from build123d import *

# Parameters (mm, degrees)
SKETCH1_R           = 37.5
BOSS_EXTRUDE1_DEPTH = 55
SKETCH2_R           = 16
CUT_EXTRUDE1_DEPTH  = 16
SKETCH3_R           = 16
CUT_EXTRUDE2_DEPTH  = 2.5
SKETCH6_R           = 8.9296875
CUT_EXTRUDE3_DEPTH  = 12.7
CUT_EXTRUDE4_START  = -15.35
SKETCH7_R           = 37.5
CUT_EXTRUDE4_DEPTH  = 15.35
SKETCH9_R           = 3.302
CUT_EXTRUDE6_DEPTH  = 67.216482087
BOSS_EXTRUDE2_START = 10
SKETCH10_R          = 37.5
SKETCH10_R_2        = 8.9296875
SKETCH10_R_3        = 3.302
BOSS_EXTRUDE2_DEPTH = 10


with BuildPart() as part:
    # Sketch1 → Boss-Extrude1 (new body)
    with BuildSketch(Plane.XY):
        Circle(SKETCH1_R)
    extrude(amount=BOSS_EXTRUDE1_DEPTH)

    # Sketch2 → Cut-Extrude1 (cut)
    with BuildSketch(Plane.XY.offset(55)):
        Circle(SKETCH2_R)
    extrude(amount=-CUT_EXTRUDE1_DEPTH, mode=Mode.SUBTRACT)

    # Sketch3 → Cut-Extrude2 (cut)
    with BuildSketch(Plane.XY.offset(39)):
        Circle(SKETCH3_R)
    extrude(amount=-CUT_EXTRUDE2_DEPTH, mode=Mode.SUBTRACT)

    # Sketch4 → Cut-Revolve1 (revolve, cut)
    with BuildSketch(Plane(origin=(0, 0, 0), x_dir=(0, 0, -1), z_dir=(1, 0, 0))):
        with BuildLine():
            Line((-12.7, 8.9281), (-12.7, 0))
            Line((-12.7, 0), (-36.5, 0))
            Line((-36.5, 0), (-36.5, 12))
            add(Edge.make_bspline(
                [(-36.5, 12), (-28.343745376, 16.523417527), (-19.165864626, 14.261468976), (-12.7, 8.9281)],
                knots=[0, 0, 0, 0, 1, 1, 1, 1], degree=3))
        make_face()
    revolve(axis=Axis((0, 0, 12.7), (0, 0, 1)), mode=Mode.SUBTRACT)

    # Sketch6 → Cut-Extrude3 (cut)
    with BuildSketch(Plane(origin=(0, 0, 0), x_dir=(-1, 0, 0), z_dir=(0, 0, -1))):
        Circle(SKETCH6_R)
    extrude(amount=-CUT_EXTRUDE3_DEPTH, mode=Mode.SUBTRACT)

    # Sketch7 → Cut-Extrude4 (cut)
    with BuildSketch(Plane.XY.offset(55).offset(CUT_EXTRUDE4_START)):
        Circle(SKETCH7_R)
    extrude(amount=CUT_EXTRUDE4_DEPTH, mode=Mode.SUBTRACT)

    # Sketch9 → Cut-Extrude6 (cut, through all)
    with BuildSketch(Plane(origin=(0, 0, 0), x_dir=(-1, 0, 0), z_dir=(0, 0, -1))):
        with Locations((0, -27.5)):
            Circle(SKETCH9_R)
        with Locations((-19.445436483, -19.445436483)):
            Circle(SKETCH9_R)
        with Locations((-27.5, 0)):
            Circle(SKETCH9_R)
        with Locations((-19.445436483, 19.445436483)):
            Circle(SKETCH9_R)
        with Locations((0, 27.5)):
            Circle(SKETCH9_R)
        with Locations((19.445436483, 19.445436483)):
            Circle(SKETCH9_R)
        with Locations((27.5, 0)):
            Circle(SKETCH9_R)
        with Locations((19.445436483, -19.445436483)):
            Circle(SKETCH9_R)
    extrude(amount=-CUT_EXTRUDE6_DEPTH, mode=Mode.SUBTRACT)

    # Sketch10 → Boss-Extrude2 (add)
    with BuildSketch(Plane(origin=(0, 0, 0), x_dir=(-1, 0, 0), z_dir=(0, 0, -1)).offset(BOSS_EXTRUDE2_START)):
        Circle(SKETCH10_R)
        Circle(SKETCH10_R_2, mode=Mode.SUBTRACT)
        with Locations((-27.5, 0)):
            Circle(SKETCH10_R_3, mode=Mode.SUBTRACT)
        with Locations((-19.445436483, -19.445436483)):
            Circle(SKETCH10_R_3, mode=Mode.SUBTRACT)
        with Locations((0, -27.5)):
            Circle(SKETCH10_R_3, mode=Mode.SUBTRACT)
        with Locations((19.445436483, -19.445436483)):
            Circle(SKETCH10_R_3, mode=Mode.SUBTRACT)
        with Locations((27.5, 0)):
            Circle(SKETCH10_R_3, mode=Mode.SUBTRACT)
        with Locations((19.445436483, 19.445436483)):
            Circle(SKETCH10_R_3, mode=Mode.SUBTRACT)
        with Locations((0, 27.5)):
            Circle(SKETCH10_R_3, mode=Mode.SUBTRACT)
        with Locations((-19.445436483, 19.445436483)):
            Circle(SKETCH10_R_3, mode=Mode.SUBTRACT)
    extrude(amount=-BOSS_EXTRUDE2_DEPTH)


solid = part.part
For this review, take the finished solid that the model builds, in its own axes (mm). Round coordinates to 2 decimals unless told otherwise and drop trailing zeros. Write each loop counter-clockwise with the first axis right and the second up, starting at its lowest first coordinate (ties: lowest second). Pieces come first, ordered by that corner, then holes. Notation, with made-up numbers: M -20,-29 L 6,-29 A13 cw 6,-20 Z; hole C 63.25,55.5 d5. An arc over 180 degrees is marked long. Write item = value, one per line. Start each with the question number.
(1) Clearance check with flat-ended pins moving along their axes: pin 1 Ø4 at (y, z) = (-16.5, 15) entering from -X; pin 2 Ø16 at (x, y) = (-6.5, -2) entering from +Z; pin 3 Ø1.5 at (x, z) = (-19, 24) entering from -Y. State where each tip first meets the part, or that it passes through.
(2) For line 1 along Y through (x, z) = (0, 37); line 2 along Y through (x, z) = (-21.5, 10); line 3 along Y through (x, z) = (-19.5, 4.5), list the stretches that pass through material, from the lowest coordinate up.
(3) We need section A-A (x = -27.5). Give the boundary of the cut face in (y, z).
(4) We need section B-B (z = 10). Give the number of separate pieces and of enclosed holes in the cut face, then the cut area to 3 significant figures.
(5) The part is to be moulded in two halves that separate along X. For faces 1 (the face through (-8, -8, -10)), 2 (the face through (6, 11, 36.5)), 3 (the face through (-3.47, -15.62, 38.1)), say which applies: +X half, -X half, draft (parallel to the pull), parting line (faces both ways), or undercut.
Results found:
q1.pin_1 = -34.58
q1.pin_2 = 36.5
q1.pin_3 = -32.76
q2.line_1 = -37.5 to -30.8, -24.2 to -16, 16 to 24.2, 30.8 to 37.5
q2.line_2 = -30.72 to -22.03, -16.86 to 16.86, 22.03 to 30.72
q2.line_3 = -32.03 to -22.75, -16.14 to 16.14, 22.75 to 32.03
q3.outline = M -25.5,-10 L -3.3,-10 L -3.3,39.65 L -25.5,39.65 Z; M 3.3,-10 L 25.5,-10 L 25.5,39.65 L 3.3,39.65 Z
q4.separate_pieces = 1
q4.enclosed_holes = 9
q4.area = 3,890 mm²
q5.face_1 = draft
q5.face_2 = undercut
q5.face_3 = undercut
